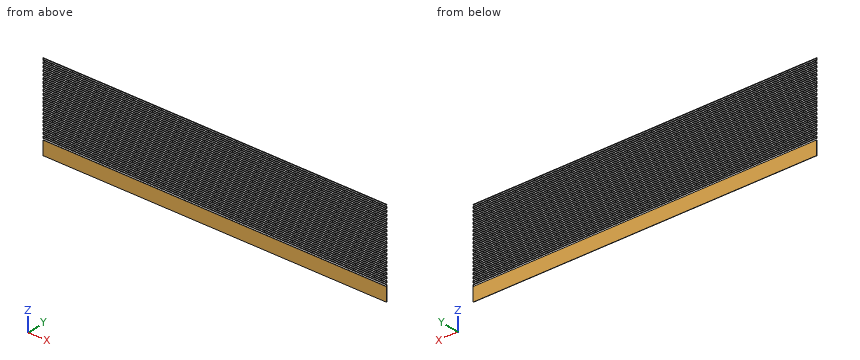
from build123d import *

# Parameters (mm, degrees)
SKETCH1_W           = 200
SKETCH1_H           = 8
BOSS_EXTRUDE1_DEPTH = 0.2
EXTRUDE_THIN1_DEPTH = 0.2
LPATTERN1_COUNT     = 21
LPATTERN1_PITCH     = 2


with BuildPart() as part:
    # Sketch1 → Boss-Extrude1 (new body)
    with BuildSketch(Plane(origin=(0, 0, 0), x_dir=(1, 0, 0), z_dir=(0, 1, 0))):
        with Locations((100, 4)):
            Rectangle(SKETCH1_W, SKETCH1_H)
    extrude(amount=BOSS_EXTRUDE1_DEPTH)

    # Sketch2 → Extrude-Thin1 (add)
    with BuildSketch(Plane(origin=(0, 0, 0), x_dir=(1, 0, 0), z_dir=(0, 1, 0))):
        Polygon((199.9, 0), (199.9, -0.9), (-0.1, -0.9), (-0.1, -2.1), (200, -2.1), (200, -1.9), (0.1, -1.9), (0.1, -1.1), (200.1, -1.1), (200.1, 0), align=None)
    extrude_thin1 = extrude(amount=EXTRUDE_THIN1_DEPTH)

    # LPattern1: Extrude-Thin1 ×21
    with Locations(*[(0, 0, i * LPATTERN1_PITCH) for i in range(1, LPATTERN1_COUNT)]):
        add(extrude_thin1)


solid = part.part
Input: part model. Units: mm. Frame: model coordinates. Round coordinates to 2 decimals unless told otherwise and drop trailing zeros.
1) Contact query for a flat-ended pin moving along its axis: P1, Ø6, axis at x = 64, z = 34.5, coming from the -Y side. Output: stop coordinate, or through.
2) Cut plane A-A (x = 134). Count the separate pieces of the cut face and the enclosed holes in it, then the cut area to 3 significant figures.
3) Ray query, L1, parallel to X at y = 0.1, z = -2; L2, parallel to X at y = 0.15, z = 17.5. Return the intervals inside material, ascending.
Geometry says:
1. P1: stops at y = 0
2. separate pieces: 43
2. enclosed holes: 0
2. area: 3.28 mm2
3. L1: x = 0 to 200
3. L2: x = -0.1 to 0.1
